from build123d import *

# Parameters (mm, degrees)
SKETCH_1_W          = 33
SKETCH_1_H          = 5
SKETCH_1_W_2        = 13
SKETCH_1_H_2        = 11.5
EXTRUDE_1_DEPTH     = 15
SKETCH_2_R          = 1.65
CUT_EXTRUDE_1_DEPTH = 26.089838581
CUT_EXTRUDE_3_DEPTH = 2
FILLET_2_R          = 0.3
FILLET_3_R          = 0.3
FILLET_4_R          = 3


with BuildPart() as part:
    # ｽｹｯﾁ1 → ﾎﾞｽ - 押し出し1 (new body)
    with BuildSketch(Plane.XY):
        Rectangle(SKETCH_1_W, SKETCH_1_H)
        with Locations((0, 8.25)):
            Rectangle(SKETCH_1_W_2, SKETCH_1_H_2)
    extrude(amount=EXTRUDE_1_DEPTH)

    # ｽｹｯﾁ2 → ｶｯﾄ - 押し出し1 (cut, through all)
    with BuildSketch(Plane(origin=(0, 2.5, 0), x_dir=(1, 0, 0), z_dir=(0, 1, 0))):
        with Locations(Location((-11.5, -10, 0), (0, 0, 180))):
            Circle(SKETCH_2_R)
        with Locations((11.5, -10)):
            Circle(SKETCH_2_R)
    extrude(amount=-CUT_EXTRUDE_1_DEPTH, mode=Mode.SUBTRACT)

    # ｽｹｯﾁ3 → ｶｯﾄ - 押し出し3 (cut)
    with BuildSketch(Plane(origin=(0, 14, 0), x_dir=(1, 0, 0), z_dir=(0, 1, 0))):
        with BuildLine():
            Line((-5.728219619, -5), (5.728219619, -5))
            ThreePointArc((5.728219619, -5), (0, -1.25), (-5.728219619, -5))
        make_face()
        with BuildLine():
            ThreePointArc((-5.728219619, -10), (0, -13.75), (5.728219619, -10))
            Line((5.728219619, -10), (-5.728219619, -10))
        make_face()
        with BuildLine():
            ThreePointArc((6.25, -7.5), (6.118164456, -6.223064727), (5.728219619, -5))
            Line((5.728219619, -5), (-5.728219619, -5))
            ThreePointArc((-5.728219619, -5), (-6.25, -7.5), (-5.728219619, -10))
            Line((-5.728219619, -10), (5.728219619, -10))
            ThreePointArc((5.728219619, -10), (6.118164456, -8.776935273), (6.25, -7.5))
        make_face()
        with BuildLine():
            ThreePointArc((-5.728219619, -10), (-6.25, -7.5), (-5.728219619, -5))
            Line((-5.728219619, -5), (-6.5, -5))
            Line((-6.5, -5), (-6.5, -10))
            Line((-6.5, -10), (-5.728219619, -10))
        make_face()
        with BuildLine():
            Line((6.5, -10), (6.5, -5))
            Line((6.5, -5), (5.728219619, -5))
            ThreePointArc((5.728219619, -5), (6.118164456, -6.223064727), (6.25, -7.5))
            ThreePointArc((6.25, -7.5), (6.118164456, -8.776935273), (5.728219619, -10))
            Line((5.728219619, -10), (6.5, -10))
        make_face()
    extrude(amount=-CUT_EXTRUDE_3_DEPTH, mode=Mode.SUBTRACT)

    # ﾌｨﾚｯﾄ2
    fillet_2_edges = [part.edges().sort_by_distance(p)[0] for p in [
        (-5.728219619, 13, 5),
        (5.728219619, 13, 5),
        (6.5, 13, 5),
        (6.5, 13, 10),
        (5.728219619, 13, 10),
        (-5.728219619, 13, 10),
        (-6.5, 13, 10),
        (-6.5, 13, 5),
    ]]
    fillet(fillet_2_edges, radius=FILLET_2_R)

    # ﾌｨﾚｯﾄ3
    fillet_3_edges = [part.edges().sort_by_distance(p)[0] for p in [
        (-6.5, 2.5, 7.5),
        (6.5, 2.5, 7.5),
    ]]
    fillet(fillet_3_edges, radius=FILLET_3_R)

    # ﾌｨﾚｯﾄ4
    fillet_4_edges = [part.edges().sort_by_distance(p)[0] for p in [
        (-16.5, 0, 0),
        (-16.5, 0, 15),
        (16.5, 0, 15),
        (16.5, 0, 0),
    ]]
    fillet(fillet_4_edges, radius=FILLET_4_R)


solid = part.part
Geometry: final body of the model. Coordinates: model frame, mm. A direction names the side the tool comes from. Give positions to 0.01 mm unless a question says otherwise; leave off trailing zeros. Loops run counter-clockwise (first coordinate to the right, second up) from the corner with the lowest first, then second, coordinate; pieces in that order, holes last. Notation, with made-up numbers: M -26,10 L -16,10 A4 ccw -16,17 Z; hole C 79,73 d5. An arc over 180 degrees is marked long. Put each result on its own line as item: value.
1) Mould query, pull axis X, two halves, no side actions, for faces 6 (the cylindrical face through (15.6, 0.04, 0.86)), 7 (the flat face through (-16.5, 0, 7)), 8 (the flat face through (12, 2.5, 7)), 9 (the cylindrical face through (0.1, 13.01, 1.25)). Classes: released by +X, released by -X, zero draft, split by the parting line, or undercut.
Computed values:
face 6: released by +X
face 7: released by -X
face 8: zero draft
face 9: undercut
2) Reachability of faces 1 (the flat face through (0, -2.5, 7)), 2 (the flat face through (-6.5, 8, 7)), 3 (the cylindrical face through (-0.1, 13.01, 13.75)), 4 (the flat face through (6.5, 8, 7)), 5 (the cylindrical face through (-15.6, 0.04, 0.86)) from +Z, -Z, +X, -X, +Y, -Y: full face, straight path, thin tool, end or side. Return the list, or none.
Computed values:
face 1: +Z, -Z, +X, -X, -Y
face 2: +Z, -Z, -X, +Y
face 3: +Y
face 4: +Z, -Z, +X, +Y
face 5: -Z, -X, +Y, -Y
3) Cut plane C-C, the plane y = 0.75. Return the cut outline in (x, z), plus the area to 3 significant figures.
Computed values:
outline: M -16.5,3 A3 ccw -13.5,0 L 13.5,0 A3 ccw 16.5,3 L 16.5,12 A3 ccw 13.5,15 L -13.5,15 A3 ccw -16.5,12 Z; hole C -11.5,10 d3.3; hole C 11.5,10 d3.3
area: 470 mm^2
4) First-contact query: P1, Ø3, axis at x = -11.5, z = 10, coming from the -Y side; P2, Ø4, axis at y = 10, z = 10.5, coming from the -X side; P3, Ø9, axis at y = 9, z = 9.5, coming from the +X side; P4, Ø3, axis at x = -10, z = 4, coming from the +Y side. Flat tips, straight axial feed; report the tip coordinate or a pass-through.
Computed values:
P1: passes through
P2: stops at x = -6.5
P3: stops at x = 6.5
P4: stops at y = 2.5
5) Cut plane B-B, the plane x = -11.5. Return the cut outline in (y, z).
Computed values:
outline: M -2.5,0 L 2.5,0 L 2.5,8.35 L -2.5,8.35 Z; M -2.5,11.65 L 2.5,11.65 L 2.5,15 L -2.5,15 Z
6) Material intervals for L1, parallel to Z at x = 11.5, y = 1.55; L2, parallel to Y at x = 3, z = 12.25; L3, parallel to Y at x = 10, z = 0.5, sorted ascending. Write a range as from..to.
Computed values:
L1: z = 0..8.35, 11.65..15
L2: y = -2.5..12
L3: y = -2.5..2.5
7) Cut plane A-A, the plane z = 7.75. Return the cut outline in (x, y), plus the area to 3 significant figures.
Computed values:
outline: M -16.5,-2.5 L 16.5,-2.5 L 16.5,2.5 L 6.8,2.5 A0.3 cw 6.5,2.8 L 6.5,12 L -6.5,12 L -6.5,2.8 A0.3 cw -6.8,2.5 L -16.5,2.5 Z
area: 289 mm^2
8) Cut plane D-D, the plane z = 11.25. Return the cut outline in (x, y), plus the area to 3 significant figures.
Computed values:
outline: M -16.5,-2.5 L -12.58,-2.5 L -12.58,2.5 L -16.5,2.5 Z; M -10.42,-2.5 L 10.42,-2.5 L 10.42,2.5 L 6.8,2.5 A0.3 cw 6.5,2.8 L 6.5,14 L 5,14 L 5,12 L -5,12 L -5,14 L -6.5,14 L -6.5,2.8 A0.3 cw -6.8,2.5 L -10.42,2.5 Z; M 12.58,-2.5 L 16.5,-2.5 L 16.5,2.5 L 12.58,2.5 Z
area: 273 mm^2
